Geometry: final body of the model. Coordinates: model frame, mm. A direction names the side the tool comes from. Give positions to 0.01 mm unless a question says otherwise; leave off trailing zeros. Loops run counter-clockwise (first coordinate to the right, second up) from the corner with the lowest first, then second, coordinate; pieces in that order, holes last. Notation, with made-up numbers: (-12.75, 83) -> (-3.75, 83) arc R26 cw to (-3.75, 100) -> close; hole circle Ø5 at (57, 3). An arc over 180 degrees is marked (long way). One line per question, with ' | ' between items. Start each with the question number.
Item 1: Mould query, pull axis X, two halves, no side actions, for faces 1 (the flat face through (-29, 1, -25.799)), 2 (the flat face through (-3, 1, 24.451)). Classes: released by +X, released by -X, zero draft, split by the parting line, or undercut.
Item 2: Section C-C on y = 1.9. Give the number of separate pieces and of enclosed holes in the cut face, then the cut area to 3 significant figures.
Item 3: Section B-B on z = 3. Return loops of the section in (x, y).
Item 4: Pin query (flat end, axial travel): P1, Ø1.5, axis at x = 28.5, y = 1, coming from the +Z side. Return the tip coordinate at first contact, or that it passes through.
Item 5: Material intervals for line 1 along Z through (x, y) = (-30, 2.7); line 2 along Z through (x, y) = (29.5, 0.75); line 3 along X through (y, z) = (1.1, -22.5), sorted ascending. Write a range as [from, to].
Item 6: Section A-A on x = 25. Return loops of the section in (y, z), then the cut area to 4 significant figures.
Item 7: Set-up query: faces 3 (the flat face through (-22, 1, -19.799)), 4 (the flat face through (29, 1, -25.799)), 5 (the flat face through (27.25, 1, 20)). Return all of +Z, -Z, +X, -X, +Y, -Y with unobstructed straight access to the full face (end or side cutting, diameter ignored); none if empty.
from build123d import *

# Parameters (mm, degrees)
SKETCH_3_W          = 66
SKETCH_3_H          = 60
EXTRUDE_1_DEPTH     = 3
SKETCH_1_W          = 3.5
SKETCH_1_H          = 10.5
SKETCH_1_H_2        = 9.75
SKETCH_1_H_3        = 4.5
SKETCH_1_W_2        = 15.25
SKETCH_1_H_4        = 3.5
SKETCH_1_W_3        = 10.5
CUT_EXTRUDE_1_DEPTH = 49.597691494


with BuildPart() as part:
    # Эскиз3 → Бобышка-Вытянуть1 (new body)
    with BuildSketch(Plane(origin=(0, 0, 0), x_dir=(1, 0, 0), z_dir=(0, 1, 0))):
        with Locations((0, 5.54905932)):
            Rectangle(SKETCH_3_W, SKETCH_3_H)
    extrude(amount=EXTRUDE_1_DEPTH)

    # Эскиз1 → Вырез-Вытянуть1 (cut, through all)
    with BuildSketch(Plane(origin=(0, 0, 0), x_dir=(1, 0, 0), z_dir=(0, 1, 0))):
        with Locations((-29, 5.54905932)):
            Rectangle(SKETCH_1_W, SKETCH_1_H)
        Polygon((-30.75, 25.79905932), (-27.25, 25.79905932), (-27.25, 23.29905932), (-17.25, 23.29905932), (-17.25, 19.79905932), (-27.25, 19.79905932), (-27.25, 15.29905932), (-30.75, 15.29905932), align=None)
        with Locations((-29, -9.45094068)):
            Rectangle(SKETCH_1_W, SKETCH_1_H)
        with Locations((29, -19.57594068)):
            Rectangle(SKETCH_1_W, SKETCH_1_H_2)
        with Locations((29, 13.04905932)):
            Rectangle(SKETCH_1_W, SKETCH_1_H_3)
        with Locations((29, -1.95094068)):
            Rectangle(SKETCH_1_W, SKETCH_1_H_3)
        with Locations((29, 30.67405932)):
            Rectangle(SKETCH_1_W, SKETCH_1_H_2)
        with Locations((-0.125, 21.54905932)):
            Rectangle(SKETCH_1_W_2, SKETCH_1_H_4)
        with Locations((22.25, 21.54905932)):
            Rectangle(SKETCH_1_W_3, SKETCH_1_H_4)
    extrude(amount=CUT_EXTRUDE_1_DEPTH, mode=Mode.SUBTRACT)


solid = part.part
Result sheet:
1) face 1: undercut | face 2: zero draft
2) separate pieces: 1 | enclosed holes: 7 | area: 3,620 mm²
3) outline: (-33, 0) -> (27.25, 0) -> (27.25, 3) -> (-33, 3) -> close; (30.75, 0) -> (33, 0) -> (33, 3) -> (30.75, 3) -> close
4) P1: stops at z = 14.7
5) line 1: z = [-35.55, -25.8], [-15.3, -10.8], [-0.3, 4.2], [14.7, 24.45] | line 2: z = [-25.8, -15.3], [-10.8, -0.3], [4.2, 14.7] | line 3: x = [-33, -30.75], [-17.25, -7.75], [7.5, 17], [27.5, 33]
6) outline: (0, -35.55) -> (3, -35.55) -> (3, -23.3) -> (0, -23.3) -> close; (0, -19.8) -> (3, -19.8) -> (3, 24.45) -> (0, 24.45) -> close | area: 169.5 mm²
7) face 3: +Y, -Y | face 4: -Z, +Y, -Y | face 5: +Z, +Y, -Y
